Input: part model. Units: mm. Frame: model coordinates. A direction names the side the tool comes from. Coordinates: 2 decimals unless noted, no trailing zeros. Loops run counter-clockwise (first coordinate to the right, second up) from the corner with the lowest first, then second, coordinate; pieces in that order, holes last.
(1) Set-up query: faces 1 (the face through (13.902, 3.451, 3.255)), 2 (the face through (16.7, 7, -2.2)), 3 (the face through (19, 0, -2)). Return all of +Z, -Z, +X, -X, +Y, -Y with unobstructed straight access to the full face (end or side cutting, diameter ignored); none if empty.
(2) Section C-C, the plane x = -49. Return loops of the section in (y, z), then the cut area to 3 significant figures.
(3) Section A-A, the plane y = -53. Return loops of the section in (x, z).
(4) Section B-B, the plane z = -4.75. Return loops of the section in (x, y).
(5) Mould query, pull axis Y, two halves, no side actions, for faces 4 (the face through (-13.902, 46.451, 3.255)), 5 (the face through (-55.732, -56.695, -10.935)), 6 (the face through (18, 50, -2)). Classes: released by +Y, released by -Y, zero draft, split by the parting line, or undercut.
(6) Line query: L1, parallel to Y at x = -98, z = -10; L2, parallel to X at y = 14, z = -4.25; L3, parallel to Y at x = -72, z = -8.75. Output: solid intervals per line, ascending.
(7) Section D-D, the plane z = 5.5. Return loops of the section in (x, y), then the cut area to 3 significant figures.
(8) Contact query for flat-ended pins moving along their axis: P1, Ø2.5, axis at x = 78.01, y = -96.05, coming from the +Z side; P2, Ø2, axis at x = 58.5, z = -9, coming from the -Y side; P3, Ø3.5, axis at x = -96.64, y = -41.95, coming from the +Z side; P4, Ø2, axis at y = 40.5, z = -5, coming from the -X side. Output: stop coordinate, or through.
```python
from build123d import *

# Parameters (mm, degrees)
BOSS_EXTRUDE2_DEPTH     = 7
CUT_EXTRUDE2_DEPTH      = 30.130224853
CUT_EXTRUDE2_DEPTH_BACK = 30.130224853
SKETCH3_R               = 2
BOSS_EXTRUDE3_DEPTH     = 36
SKETCH5_R               = 2
BOSS_EXTRUDE4_DEPTH     = 7
SKETCH13_W              = 49.8
SKETCH13_H              = 5
BOSS_EXTRUDE6_DEPTH     = 12.25
SKETCH15_W              = 49.8
SKETCH15_H              = 5
BOSS_EXTRUDE7_DEPTH     = 30
SKETCH12_R              = 1.5
SKETCH12_R_2            = 2.625
BOSS_EXTRUDE8_DEPTH     = 5


with BuildPart() as part:
    # Sketch1 → Boss-Extrude2 (new body)
    with BuildSketch(Plane(origin=(0, 0, 0), x_dir=(1, 0, 0), z_dir=(0, 1, 0))):
        with BuildLine():
            Line((-24.9, 0), (-24.9, 13.4))
            Line((-24.9, 13.4), (24.9, 13.4))
            Line((24.9, 13.4), (24.9, 0))
            ThreePointArc((24.9, 0), (23.392904185, -4.800819919), (19.412411454, -7.878950407))
            Line((19.412411454, -7.878950407), (8.235013612, 1.5))
            ThreePointArc((8.235013612, 1.5), (11.116692467, 6.448255578), (16.5, 8.4))
            Line((16.5, 8.4), (-16.5, 8.4))
            ThreePointArc((-16.5, 8.4), (-11.116692467, 6.448255578), (-8.235013612, 1.5))
            Line((-8.235013612, 1.5), (-19.412411454, -7.878950407))
            ThreePointArc((-19.412411454, -7.878950407), (-23.392904185, -4.800819919), (-24.9, 0))
        make_face()
    extrude(amount=BOSS_EXTRUDE2_DEPTH)

    # Sketch3 → Cut-Extrude2 (cut, two sides: drawn at the far end of the back side and taken through both)
    with BuildSketch(Plane(origin=(0, 7, 0), x_dir=(1, 0, 0), z_dir=(0, 1, 0)).offset(-CUT_EXTRUDE2_DEPTH_BACK)):
        with Locations(Location((-16.5, 0, 0), (0, 0, 270))):
            Circle(SKETCH3_R)
        with Locations(Location((16.5, 0, 0), (0, 0, 270))):
            Circle(SKETCH3_R)
    extrude(amount=CUT_EXTRUDE2_DEPTH + CUT_EXTRUDE2_DEPTH_BACK, mode=Mode.SUBTRACT)

    # Sketch4 → Boss-Extrude3 (add)
    with BuildSketch(Plane(origin=(0, 7, 0), x_dir=(1, 0, 0), z_dir=(0, 1, 0))):
        Polygon((-24.9, 13.4), (-24.9, 0), (-20.9, 0), (-20.9, 8.4), (-16.5, 8.4), (16.5, 8.4), (20.9, 8.4), (20.9, 0), (24.9, 0), (24.9, 13.4), align=None)
    extrude(amount=BOSS_EXTRUDE3_DEPTH)

    # Sketch5 → Boss-Extrude4 (add)
    with BuildSketch(Plane(origin=(0, 43, 0), x_dir=(1, 0, 0), z_dir=(0, 1, 0))):
        with BuildLine():
            Line((-24.9, 13.4), (-24.9, 0))
            ThreePointArc((-24.9, 0), (-23.392904185, -4.800819919), (-19.412411454, -7.878950407))
            Line((-19.412411454, -7.878950407), (-8.235013612, 1.5))
            ThreePointArc((-8.235013612, 1.5), (-11.116692467, 6.448255578), (-16.5, 8.4))
            Line((-16.5, 8.4), (16.5, 8.4))
            ThreePointArc((16.5, 8.4), (11.116692467, 6.448255578), (8.235013612, 1.5))
            Line((8.235013612, 1.5), (19.412411454, -7.878950407))
            ThreePointArc((19.412411454, -7.878950407), (23.392904185, -4.800819919), (24.9, 0))
            Line((24.9, 0), (24.9, 13.4))
            Line((24.9, 13.4), (-24.9, 13.4))
        make_face()
        with Locations(Location((16.5, 0, 0), (0, 0, 270))):
            Circle(SKETCH5_R, mode=Mode.SUBTRACT)
        with Locations(Location((-16.5, 0, 0), (0, 0, 270))):
            Circle(SKETCH5_R, mode=Mode.SUBTRACT)
    extrude(amount=BOSS_EXTRUDE4_DEPTH)

    # Sketch13 → Boss-Extrude6 (add)
    with BuildSketch(Plane(origin=(0, 50, 0), x_dir=(1, 0, 0), z_dir=(0, 1, 0))):
        with Locations((0, 10.9)):
            Rectangle(SKETCH13_W, SKETCH13_H)
    extrude(amount=BOSS_EXTRUDE6_DEPTH)

    # Sketch15 → Boss-Extrude7 (add)
    with BuildSketch(Plane.XZ):
        with Locations((0, -10.9)):
            Rectangle(SKETCH15_W, SKETCH15_H)
    extrude(amount=BOSS_EXTRUDE7_DEPTH)

    # Sketch12 → Boss-Extrude8 (add)
    with BuildSketch(Plane(origin=(0, 0, -13.4), x_dir=(-1, 0, 0), z_dir=(0, 0, -1))):
        with BuildLine():
            Line((3.57214695, -63.566782317), (-59.47254153, -87.376896171))
            ThreePointArc((-59.47254153, -87.376896171), (-84.246316334, -103.146864291), (-55.232789428, -98.602959689))
            Line((-55.232789428, -98.602959689), (12.489425518, -73.02628246))
            Line((12.489425518, -73.02628246), (62.145671786, -125.701912707))
            ThreePointArc((62.145671786, -125.701912707), (86.23094036, -142.504640172), (70.877518071, -117.470578644))
            Line((70.877518071, -117.470578644), (24.650994329, -68.433217683))
            Line((24.650994329, -68.433217683), (87.69568281, -44.623103829))
            ThreePointArc((87.69568281, -44.623103829), (112.469457614, -28.853135709), (83.455930708, -33.397040311))
            Line((83.455930708, -33.397040311), (15.733715762, -58.97371754))
            Line((15.733715762, -58.97371754), (-33.922530506, -6.298087293))
            ThreePointArc((-33.922530506, -6.298087293), (-58.00779908, 10.504640172), (-42.654376791, -14.529421356))
            Line((-42.654376791, -14.529421356), (3.57214695, -63.566782317))
        make_face()
        with Locations((-49.518239937, -8.205128203)):
            Circle(SKETCH12_R, mode=Mode.SUBTRACT)
        with Locations((-55.51359202, 1.38944075)):
            Circle(SKETCH12_R, mode=Mode.SUBTRACT)
        with Locations((-45.919023067, 7.384792833)):
            Circle(SKETCH12_R, mode=Mode.SUBTRACT)
        with Locations((-39.923670984, -2.20977612)):
            Circle(SKETCH12_R, mode=Mode.SUBTRACT)
        with Locations(Location((-62.418776418, -99.646782598, 0), (0, 0, 180))):
            Circle(SKETCH12_R, mode=Mode.SUBTRACT)
        with Locations(Location((-72.013345371, -105.642134682, 0), (0, 0, 180))):
            Circle(SKETCH12_R, mode=Mode.SUBTRACT)
        with Locations(Location((-68.414128501, -90.052213645, 0), (0, 0, 180))):
            Circle(SKETCH12_R, mode=Mode.SUBTRACT)
        with Locations(Location((-78.008697455, -96.047565729, 0), (0, 0, 180))):
            Circle(SKETCH12_R, mode=Mode.SUBTRACT)
        with Locations(Location((100.236486651, -26.357865318, 0), (0, 0, 180))):
            Circle(SKETCH12_R, mode=Mode.SUBTRACT)
        with Locations(Location((90.641917698, -32.353217402, 0), (0, 0, 180))):
            Circle(SKETCH12_R, mode=Mode.SUBTRACT)
        with Locations(Location((96.637269781, -41.947786355, 0), (0, 0, 180))):
            Circle(SKETCH12_R, mode=Mode.SUBTRACT)
        with Locations(Location((106.231838734, -35.952434271, 0), (0, 0, 180))):
            Circle(SKETCH12_R, mode=Mode.SUBTRACT)
        with Locations((68.146812263, -129.79022388)):
            Circle(SKETCH12_R, mode=Mode.SUBTRACT)
        with Locations((77.741381216, -123.794871797)):
            Circle(SKETCH12_R, mode=Mode.SUBTRACT)
        with Locations((83.7367333, -133.38944075)):
            Circle(SKETCH12_R, mode=Mode.SUBTRACT)
        with Locations((74.142164347, -139.384792833)):
            Circle(SKETCH12_R, mode=Mode.SUBTRACT)
        with Locations((-47.718631502, -0.410167685)):
            Circle(SKETCH12_R_2, mode=Mode.SUBTRACT)
        with Locations(Location((-70.213736936, -97.847174163, 0), (0, 0, 180))):
            Circle(SKETCH12_R_2, mode=Mode.SUBTRACT)
        with Locations(Location((98.436878216, -34.152825837, 0), (0, 0, 180))):
            Circle(SKETCH12_R_2, mode=Mode.SUBTRACT)
        with Locations((75.941772782, -131.589832315)):
            Circle(SKETCH12_R_2, mode=Mode.SUBTRACT)
    extrude(amount=-BOSS_EXTRUDE8_DEPTH)


solid = part.part
```
Report:
1. face 1: +Z, +Y, -Y
1. face 2: +Z
1. face 3: +Z, +X, -X, -Y
2. outline: (-111.76, -13.4) - (-94.26, -13.4) - (-94.26, -8.4) - (-111.76, -8.4) - close; (-59.24, -13.4) - (-46.41, -13.4) - (-46.41, -8.4) - (-59.24, -8.4) - close
2. area: 152 mm2
3. outline: (-65.52, -13.4) - (-31.55, -13.4) - (-31.55, -8.4) - (-65.52, -8.4) - close; (-10.1, -13.4) - (6.39, -13.4) - (6.39, -8.4) - (-10.1, -8.4) - close
4. outline: (-24.9, 0) - (-9.57, 0) - (-9.57, 7) - (-20.9, 7) - (-20.9, 43) - (-9.57, 43) - (-9.57, 50) - (-24.9, 50) - close; (9.57, 0) - (24.9, 0) - (24.9, 50) - (9.57, 50) - (9.57, 43) - (20.9, 43) - (20.9, 7) - (9.57, 7) - close
5. face 4: zero draft
5. face 5: undercut
5. face 6: released by +Y
6. L1: y = -49.15 to -42.57, -41.32 to -36.74, -31.56 to -19.16
6. L2: x = -24.9 to -20.9, 20.9 to 24.9
6. L3: y = -146.06 to -117.12, -50.55 to -37.72
7. outline: (-22.85, 0) - (-16.58, 0) - (-16.58, 7) - (-22.85, 7) - close; (-22.85, 43) - (-16.58, 43) - (-16.58, 50) - (-22.85, 50) - close; (16.58, 0) - (22.85, 0) - (22.85, 7) - (16.58, 7) - close; (16.58, 43) - (22.85, 43) - (22.85, 50) - (16.58, 50) - close
7. area: 176 mm2
8. P1: passes through
8. P2: stops at y = -108.35
8. P3: stops at z = -8.4
8. P4: stops at x = -24.9
